Autodesk Inventor part; units mm, degrees
ref_plane "YZ Plane" through (0, 0, 0) normal (1, 0, 0) x (0, 1, 0)
ref_plane "XY Plane" through (0, 0, 0) normal (0, 0, 1) x (1, 0, 0)
sketch "Sketch1" plane through (0, 0, 0) normal (0, 1, 0) x (-1, 0, 0)
  circle A0 centre (0, 0) radius 10
  circle A1 centre (0, 0) radius 12.5
  line L0 (12.5, 0) -> (12.5, 50)
  line L1 (-12.5, 0) -> (-12.5, 50)
  line L2 (-12.5, 50) -> (12.5, 50)
  dimension "d0" = 20
  dimension "d1" = 25
  dimension "d2" = 50
extrude "Extrusion1" add sketch "Sketch1" along normal blind 15
sketch "Sketch2" plane through (-12.5, 0, 0) normal (-1, 0, 0) x (0, 0, 1)
  line L0 (-12.5, 0) -> (-12.5, 15)
  line L1 (-12.5, 7.5) -> (37.5, 7.5)
  line L2 (25, 7.5) -> (25, 4.5)
  line L3 (25, 4.5) -> (25, 10.5)
  line L4 (25, 10.5) -> (75, 10.5)
  line L5 (75, 10.5) -> (75, 4.5)
  line L6 (75, 4.5) -> (25, 4.5)
  point P0 (0, 0)
  dimension "d5" = 50
  dimension "d8" = 3
  dimension "d9" = 6
  dimension "d10" = 50
extrude "Extrusion2" add sketch "Sketch2" along normal blind 10
sketch "Sketch3" plane through (-12.5, 0, 50) normal (0, 0, 1) x (1, 0, 0)
  point P0 (12.5, 0)
sketch "Sketch4" plane through (-12.5, 0, 50) normal (0, 0, 1) x (1, 0, 0)
  line L0 (25, 0) -> (25, 15)
  line L1 (25, 0) -> (25, 15)
  line L2 (0, 15) -> (25, 15)
  line L3 (25, 15) -> (0, 15)
  line L4 (0, 0) -> (0, 15)
  line L5 (0, 15) -> (0, 0)
  line L6 (0, 0) -> (25, 0)
  line L7 (0, 0) -> (25, 0)
  point P0 (12.5, 0)
extrude "Extrusion3" add sketch "Sketch4" along normal blind 25
sketch "Sketch5" plane through (-12.5, 4.5, 25) normal (0, -1, 0) x (1, 0, 0)
  point P0 (12.5, -25)
sketch "Sketch8" plane through (-12.5, 4.5, 25) normal (0, -1, 0) x (1, 0, 0)
  line L0 (0, 0) -> (-10, 0)
  line L1 (-5, 0) -> (-5, 50)
  line L2 (0, 50) -> (-10, 50)
  line L3 (-3, 12) -> (-7, 12)
  line L4 (-7, 12) -> (-7, 8)
  line L5 (-7, 8) -> (-3, 8)
  line L6 (-3, 8) -> (-3, 12)
  line L7 (-3, 12) -> (-7, 8) construction
  line L8 (-7, 12) -> (-3, 8) construction
  line L9 (-5, 10) -> (-5, 23)
  line L10 (-7, 21) -> (-3, 21)
  line L11 (-3, 21) -> (-3, 25)
  line L12 (-3, 25) -> (-7, 25)
  line L13 (-7, 25) -> (-7, 21)
  line L14 (-7, 21) -> (-3, 25) construction
  line L15 (-3, 21) -> (-7, 25) construction
  line L16 (-5, 23) -> (-5, 36)
  line L17 (-7, 34) -> (-3, 34)
  line L18 (-3, 34) -> (-3, 38)
  line L19 (-3, 38) -> (-7, 38)
  line L20 (-7, 38) -> (-7, 34)
  line L21 (-7, 34) -> (-3, 38) construction
  line L22 (-3, 34) -> (-7, 38) construction
  point P0 (12.5, -25)
  dimension "d40" = 4
  dimension "d41" = 4
  dimension "d42" = 13
  dimension "d43" = 4
  dimension "d44" = 4
  dimension "d45" = 13
  dimension "d46" = 4
  dimension "d47" = 4
extrude "Extrusion6" cut sketch "Sketch8" against normal blind 10
sketch "Sketch9" plane through (0, 0, 0) normal (0, -1, 0) x (1, 0, 0)
  line L0 (-12.5, 25) -> (-22.5, 25)
  line L1 (-12.5, 25) -> (12.5, 25)
  line L2 (12.5, 0) -> (12.5, 75)
  line L3 (-12.5, 25) -> (-12.5, 75)
  line L4 (-12.5, 25) -> (-12.5, 75)
  line L5 (-12.5, 75) -> (12.5, 75)
  line L6 (-12.5, 75) -> (12.5, 75)
  line L7 (12.5, 75) -> (12.5, 25)
  line L8 (12.5, 0) -> (12.5, 30)
  line L9 (-12.5, 25) -> (-10.5, 25)
  line L10 (-10.5, 25) -> (-10.5, 75)
  line L11 (-12.5, 75) -> (-12.5, 25)
  line L12 (-10.5, 25) -> (12.5, 30)
  point P0 (0, 0)
  dimension "d50" = 30
  dimension "d51" = 2
extrude "Extrusion7" add sketch "Sketch9" along normal blind 13 contours L10 L5 L2 L12
sketch "Sketch10" plane through (0, -13, 0) normal (0, -1, 0) x (1, 0, 0)
  point P0 (0, 0)
sketch "Sketch11" plane through (0, -13, 0) normal (0, -1, 0) x (1, 0, 0)
  line L0 (-10.5, 25) -> (12.5, 30)
  line L1 (12.5, 30) -> (-10.5, 30)
  line L2 (-10.5, 25) -> (-10.5, 75)
  line L3 (-10.5, 30) -> (1, 30)
  line L4 (1, 30) -> (1, 75)
  line L5 (12.5, 75) -> (-12.5, 75)
  line L6 (-1, 42) -> (3, 42)
  line L7 (3, 42) -> (3, 38)
  line L8 (3, 38) -> (-1, 38)
  line L9 (-1, 38) -> (-1, 42)
  line L10 (-1, 42) -> (3, 38) construction
  line L11 (3, 42) -> (-1, 38) construction
  line L12 (1, 40) -> (1, 52.5)
  line L13 (-1, 50.5) -> (3, 50.5)
  line L14 (3, 50.5) -> (3, 54.5)
  line L15 (3, 54.5) -> (-1, 54.5)
  line L16 (-1, 54.5) -> (-1, 50.5)
  line L17 (-1, 50.5) -> (3, 54.5) construction
  line L18 (3, 50.5) -> (-1, 54.5) construction
  line L19 (1, 52.5) -> (1, 65)
  line L20 (-1, 63) -> (3, 63)
  line L21 (3, 63) -> (3, 67)
  line L22 (3, 67) -> (-1, 67)
  line L23 (-1, 67) -> (-1, 63)
  line L24 (-1, 63) -> (3, 67) construction
  line L25 (3, 63) -> (-1, 67) construction
  line L26 (-1, 38) -> (-1, 42)
  line L27 (-1, 38) -> (3, 38)
  line L28 (3, 38) -> (3, 42)
  line L29 (3, 42) -> (-1, 42)
  line L30 (-1, 42) -> (-1, 38)
  line L31 (-1, 38) -> (3, 42) construction
  line L32 (3, 38) -> (-1, 42) construction
  point P0 (0, 0)
  dimension "d54" = 11.5
  dimension "d55" = 4
  dimension "d56" = 4
  dimension "d57" = 12.5
  dimension "d58" = 4
  dimension "d59" = 4
  dimension "d60" = 12.5
  dimension "d61" = 4
  dimension "d62" = 4
extrude "Extrusion8" cut sketch "Sketch11" against normal blind 50 contours L8 L9 L6 L4 | L4 L6 L7 L8 | L22 L21 L20 L4 | L4 L20 L23 L22 | L13 L16 L15 L4 | L4 L15 L14 L13
ref_plane "Work Plane1" through (0, 7.5, 0) normal (0, 1, 0) x (-1, 0, 0)
mirror "Mirror1" about plane through (0, 7.5, 0) normal (0, 1, 0) of "Extrusion7"
mirror "Mirror2" about plane through (0, 7.5, 0) normal (0, 1, 0) of "Extrusion8"
sketch "Sketch12" plane through (-22.5, 0, 0) normal (-1, 0, 0) x (0, 0, 1)
  point P0 (0, 0)
sketch "Sketch13" plane through (-12.5, 4.5, 25) normal (0, -1, 0) x (1, 0, 0)
  point P0 (12.5, -25)
sketch "Sketch14" plane through (-12.5, 4.5, 25) normal (0, -1, 0) x (1, 0, 0)
  point P0 (12.5, -25)
sketch "Sketch15" plane through (-10.5, 15, 25) normal (0.2124296, 0, -0.9771764) x (-0.9771764, 0, -0.2124296)
  line L0 (-23.5372, 0) -> (-23.5372, 13)
  line L1 (-14.7001, 13) -> (-18.6088, 13)
  line L2 (-23.5372, 0) -> (-18.5372, 0)
  line L3 (-18.5372, 0) -> (-18.5372, 13)
  line L4 (-18.5372, 13) -> (-23.5372, 13)
  line L5 (-23.5372, 13) -> (-23.5372, 0)
  line L6 (-23.5372, -28) -> (-33.0965, -28)
  line L7 (-18.6088, -28) -> (-18.6088, 13)
  line L8 (-23.5372, -28) -> (-18.6088, -28)
  line L9 (-18.6088, -28) -> (-18.6088, -15)
  line L10 (-18.6088, -15) -> (-23.5372, -15)
  line L11 (-23.5372, -15) -> (-23.5372, -28)
  point P0 (-4.9496, -15)
  point P1 (-18.6088, 0)
  dimension "d66" = 5
extrude "Extrusion9" add sketch "Sketch15" along normal blind 2 contours L0 L4 L7 L2 | L8 L11 L10 L7
sketch "Sketch16" plane through (0, 15, 0) normal (0, 1, 0) x (1, 0, 0)
  circle A0 centre (0, 0) radius 10
  circle A1 centre (0, 0) radius 12.5
  dimension "d69" = 25
extrude "Extrusion10" add sketch "Sketch16" along normal blind 2
sketch "Sketch17" plane through (0, 0, 0) normal (0, -1, 0) x (1, 0, 0)
  circle A0 centre (0, 0) radius 10
  circle A1 centre (0, 0) radius 10
  circle A2 centre (0, 0) radius 12.5
extrude "Extrusion11" add sketch "Sketch17" along normal blind 2
properties part number "Part10copycopy"
Can you work these out from the model? Positions are in its coordinate system, mm. A direction names the side the tool comes from. Give positions to 0.01 mm unless a question says otherwise; leave off trailing zeros. Write each loop counter-clockwise with the first axis right and the second up, starting at its lowest first coordinate (ties: lowest second). Pieces come first, ordered by that corner, then holes. Notation, with made-up numbers: (19.25, -2) -> (58.25, -2) arc R16 cw to (58.25, 5) -> close; hole circle Ø8 at (31, 40.25). An arc over 180 degrees is marked (long way). Write item = value, one per line.
(1) I'm going to push flat-ended pins straight in: P1, Ø2, axis at x = 6, z = 22, coming from the +Y side; P2, Ø4, axis at y = -5.5, z = 60, coming from the -X side; P3, Ø3, axis at x = -10, z = 23.5, coming from the -Y side; P4, Ø18, axis at x = 0, z = 0, coming from the -Y side. Where does each tip first touch, or does it pass through?
Worked out:
P1 = 15
P2 = -10.5
P3 = 0
P4 = through
(2) Suppose I cut it at A-A on y = 9. Count the separate pieces of the cut face and the enclosed holes in it, then the cut area to 3 significant figures.
Worked out:
separate_pieces = 1
enclosed_holes = 7
area = 2,210 mm^2
(3) For faces 4 (the face through (-17, 7, 25)), 5 (the face through (12.71, 21.41, 29.04)), 6 (the face through (-15.5, 7, 48)), which set-ups out of +Z, -Z, +X, -X, +Y, -Y let a thin tool reach every point of the face, with its end or its side?
Worked out:
face_4 = -Z, -X, +Y, -Y
face_5 = +Z, +X, +Y, -Y
face_6 = +Y, -Y
(4) I need wall thicknesses on probe 1 along Z at (x, y) = (0, 9); probe 2 along X at (y, z) = (-1.5, 0); probe 3 along Z at (x, y) = (0, 16.55). Which ranges of each line are inside material? Lowest first, please. Write a range as from..to.
Worked out:
probe_1 = -12.5..-10, 10..38, 42..50.5, 54.5..63, 67..75
probe_2 = -12.5..-10, 10..12.5
probe_3 = -12.5..-10, 10..12.5, 27.28..38, 42..50.5, 54.5..63, 67..75
(5) Thinking about a two-plate mould opening in Z: for faces 1 (the face through (-10.5, -6, 50)), 2 (the face through (12.71, -6.41, 29.04)), 3 (the face through (-15.5, 7, 61)), which applies, released by +Z, released by -Z, zero draft, split by the parting line, or undercut?
Worked out:
face_1 = zero draft
face_2 = released by +Z
face_3 = undercut
(6) Suppose I cut it at D-D on y = 3.5. Write out the boundary of the cut face in (x, z), then the cut area to 3 significant figures.
Worked out:
outline = (-12.5, 0) arc R12.5 ccw to (12.5, 0) -> (12.5, 75) -> (-12.5, 75) -> close; hole circle Ø20 at (0, 0); hole (-1, 38) -> (3, 38) -> (3, 42) -> (-1, 42) -> close; hole (-1, 50.5) -> (3, 50.5) -> (3, 54.5) -> (-1, 54.5) -> close; hole (-1, 63) -> (3, 63) -> (3, 67) -> (-1, 67) -> close
area = 1,760 mm^2
(7) Suppose I cut it at B-B on z = 62. Write out the boundary of the cut face in (x, y).
Worked out:
outline = (-22.5, 4.5) -> (-19.5, 4.5) -> (-19.5, 10.5) -> (-22.5, 10.5) -> close; (-15.5, 4.5) -> (-12.5, 4.5) -> (-12.5, 0) -> (-10.5, 0) -> (-10.5, -13) -> (12.5, -13) -> (12.5, 28) -> (-10.5, 28) -> (-10.5, 15) -> (-12.5, 15) -> (-12.5, 10.5) -> (-15.5, 10.5) -> close
(8) Suppose I cut it at C-C on x = 5.5. Write out the boundary of the cut face in (y, z).
Worked out:
outline = (-13, 28.48) -> (0, 28.48) -> (0, 11.22) -> (-2, 11.22) -> (-2, 8.35) -> (17, 8.35) -> (17, 11.22) -> (15, 11.22) -> (15, 28.48) -> (28, 28.48) -> (28, 75) -> (-13, 75) -> close; (-2, -11.22) -> (17, -11.22) -> (17, -8.35) -> (-2, -8.35) -> close
